The listing builds one solid part. Answer for the finished solid, in the listing's coordinates (mm). Face numbers are marked on the shaded views. A direction names the side the tool comes from. Give positions to 0.01 mm unless a question says otherwise; leave off trailing zeros. Order: outer loops, then holes, each group sorted by start corner. A loop starts at its lowest first (then second) coordinate and runs counter-clockwise, first axis right, second up. Notation, with made-up numbers: (-15.5, -22.5) -> (34.5, -22.5) arc R13 cw to (34.5, 0.5) -> close; hole circle Ø4 at (-2, 62). An arc over 180 degrees is marked (long way). Answer as a JSON object with one key per item and string values. Group by question number.
```python
from build123d import *

# Parameters (mm, degrees)
SKETCH_1_W           = 20
SKETCH_1_H           = 20
SKETCH_1_R           = 7.5
EXTRUDE_1_DEPTH      = 10
EXTRUDE_2_DEPTH      = 0.0001
EXTRUDE_2_DEPTH_BACK = 10
SKETCH_2_W           = 5
SKETCH_2_H           = 2
SKETCH_3_R           = 1.5
CUT_EXTRUDE_1_DEPTH  = 27.925861175
SKETCH_4_W           = 20
SKETCH_4_H           = 20
EXTRUDE_3_DEPTH      = 2
SKETCH_5_W           = 9
SKETCH_5_H           = 20
EXTRUDE_4_DEPTH      = 25
SKETCH_7_R           = 3
CUT_EXTRUDE_2_DEPTH  = 10
CUT_EXTRUDE_3_DEPTH  = 10
SKETCH_9_W           = 10.0001
SKETCH_9_H           = 5
CUT_EXTRUDE_4_DEPTH  = 45.654227124


with BuildPart() as part:
    # 草图1 → 凸台-拉伸1 (new body)
    with BuildSketch(Plane(origin=(0, 0, 0), x_dir=(0, 0, -1), z_dir=(1, 0, 0))):
        Rectangle(SKETCH_1_W, SKETCH_1_H)
        Circle(SKETCH_1_R, mode=Mode.SUBTRACT)
    extrude(amount=EXTRUDE_1_DEPTH)

    # 草图2 → 凸台-拉伸2 (add, two sides: drawn at the far end of the back side and taken through both)
    with BuildSketch(Plane(origin=(10, 0, 0), x_dir=(0, 0, -1), z_dir=(1, 0, 0)).offset(-EXTRUDE_2_DEPTH_BACK)):
        with Locations((-12.5, 9)):
            Rectangle(SKETCH_2_W, SKETCH_2_H)
        with Locations((-12.5, -9)):
            Rectangle(SKETCH_2_W, SKETCH_2_H)
        with Locations((12.5, -9)):
            Rectangle(SKETCH_2_W, SKETCH_2_H)
        with Locations((12.5, 9)):
            Rectangle(SKETCH_2_W, SKETCH_2_H)
    extrude(amount=EXTRUDE_2_DEPTH + EXTRUDE_2_DEPTH_BACK)

    # 草图3 → 切除-拉伸1 (cut, through all)
    with BuildSketch(Plane(origin=(0, 10, 0), x_dir=(1, 0, 0), z_dir=(0, 1, 0))):
        with Locations(Location((5.00005, 12.5, 0), (0, 0, 270))):
            Circle(SKETCH_3_R)
        with Locations(Location((5.00005, -12.5, 0), (0, 0, 270))):
            Circle(SKETCH_3_R)
    extrude(amount=-CUT_EXTRUDE_1_DEPTH, mode=Mode.SUBTRACT)

    # 草图4 → 凸台-拉伸3 (add)
    with BuildSketch(Plane(origin=(10, 0, 0), x_dir=(0, 0, -1), z_dir=(1, 0, 0))):
        Rectangle(SKETCH_4_W, SKETCH_4_H)
    extrude(amount=EXTRUDE_3_DEPTH)

    # 草图5 → 凸台-拉伸4 (add)
    with BuildSketch(Plane(origin=(12, 0, 0), x_dir=(0, 0, -1), z_dir=(1, 0, 0))):
        Rectangle(SKETCH_5_W, SKETCH_5_H)
    extrude(amount=EXTRUDE_4_DEPTH)

    # 草图7 → 切除-拉伸2 (cut)
    with BuildSketch(Plane(origin=(0, 0, -4.5), x_dir=(-1, 0, 0), z_dir=(0, 0, -1))):
        with Locations((-27, 0)):
            Circle(SKETCH_7_R)
    extrude(amount=-CUT_EXTRUDE_2_DEPTH, mode=Mode.SUBTRACT)

    # 草图8 → 切除-拉伸3 (cut)
    with BuildSketch(Plane(origin=(0, 0, -4.5), x_dir=(-1, 0, 0), z_dir=(0, 0, -1))):
        with BuildLine():
            Line((-37, -10), (-27, -10))
            ThreePointArc((-27, -10), (-34.071067812, -7.071067812), (-37, 0))
            Line((-37, 0), (-37, -10))
        make_face()
        with BuildLine():
            Line((-37, 10), (-37, 0))
            ThreePointArc((-37, 0), (-34.071067812, 7.071067812), (-27, 10))
            Line((-27, 10), (-37, 10))
        make_face()
    extrude(amount=-CUT_EXTRUDE_3_DEPTH, mode=Mode.SUBTRACT)

    # 草图9 → 切除-拉伸4 (cut, through all)
    with BuildSketch(Plane.XZ.offset(10)):
        with Locations((5.00005, -12.5)):
            Rectangle(SKETCH_9_W, SKETCH_9_H)
        with Locations((5.00005, 12.5)):
            Rectangle(SKETCH_9_W, SKETCH_9_H)
    extrude(amount=-CUT_EXTRUDE_4_DEPTH, mode=Mode.SUBTRACT)


solid = part.part
```
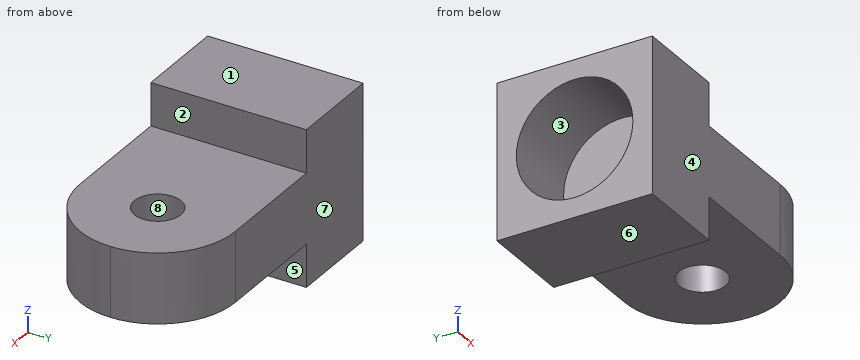
(1) Find the intervals of material crossed by line 1 along Y through (x, z) = (7, 0); line 2 along Y through (x, z) = (27, -0.25); line 3 along X through (y, z) = (6.5, -7.75), in increasing order. Write a range as [from, to].
(2) A cutting plane is placed at D-D (y = -8). Determine the outline of the cut face in (x, z), and give its area (3 significant figures).
(3) A cutting plane is placed at C-C (z = -1). Determine the outline of the cut face in (x, y).
(4) Flat-ended cylindrical pins translate along their axes: pin 1 Ø6 at (x, y) = (32, -0.5) entering from +Z; pin 2 Ø1.6 at (y, z) = (3, 7.5) entering from +X; pin 3 Ø6 at (x, y) = (16.5, -1) entering from -Z. Find the tip coordinate at first contact, or state that the pin passes through.
(5) Which of the six approach directions +Z, -Z, +X, -X, +Y, -Y give full straight-line access (tool end or side, diameter ignored) to the marked faces 1, 2, 3, 4 and 5?
(6) A cutting plane is placed at B-B (x = 6.5). Determine the outline of the cut face in (y, z), and give its area (3 significant figures).
(7) A cutting plane is placed at A-A (y = -0.75). Determine the outline of the cut face in (x, z), and give its area (3 significant figures).
(8) For a pull along Y with two mould halves and no side action, classify the marked faces 6, 7 and 8 as +Y half, -Y half, draft (parallel to the pull), parting line (faces both ways), or undercut.
Check sheet entries:
{
 "1": {"line 1": "y = [-10, -7.5], [7.5, 10]", "line 2": "y = [-10, -3], [3, 10]", "line 3": "x = [0, 12]"},
 "2": {"outline": "(0, -10) -> (12, -10) -> (12, -4.5) -> (33, -4.5) -> (33, 4.5) -> (12, 4.5) -> (12, 10) -> (0, 10) -> close", "area": "429 mm2"},
 "3": {"outline": "(0, -10) -> (27, -10) arc R10 ccw to (27, 10) -> (0, 10) -> (0, 7.43) -> (10, 7.43) -> (10, -7.43) -> (0, -7.43) -> close; hole circle Ø6 at (27, 0)"},
 "4": {"pin 1": "stops at z = 4.5", "pin 2": "stops at x = 12", "pin 3": "stops at z = -4.5"},
 "5": {"face 1": "+Z, +X, -X, +Y, -Y", "face 2": "+Z, +X, +Y, -Y", "face 3": "-X", "face 4": "+Z, -Z, +X, -X, -Y", "face 5": "-Z, +X, +Y, -Y"},
 "6": {"outline": "(-10, -10) -> (10, -10) -> (10, 10) -> (-10, 10) -> close; hole circle Ø15 at (0, 0)", "area": "223 mm2"},
 "7": {"outline": "(0, -10) -> (12, -10) -> (12, -4.5) -> (24.1, -4.5) -> (24.1, 4.5) -> (12, 4.5) -> (12, 10) -> (0, 10) -> (0, 7.46) -> (10, 7.46) -> (10, -7.46) -> (0, -7.46) -> close; (29.9, -4.5) -> (36.97, -4.5) -> (36.97, 4.5) -> (29.9, 4.5) -> close", "area": "263 mm2"},
 "8": {"face 6": "draft", "face 7": "+Y half", "face 8": "undercut"}
}
